```python
from build123d import *

# Parameters (mm, degrees)
SKETCH1_R           = 23
SKETCH1_R_2         = 14
BOSS_EXTRUDE1_DEPTH = 3.175


with BuildPart() as part:
    # Sketch1 → Boss-Extrude1 (new body)
    with BuildSketch(Plane(origin=(0, 0, 0), x_dir=(1, 0, 0), z_dir=(0, 1, 0))):
        Polygon((74.275, 82.5), (-74.275, 82.5), (-74.275, 76.15), (-144.275, 76.15), (-144.275, 82.5), (-225, 82.5), (-225, 35), (-218.65, 35), (-218.65, -35), (-225, -35), (-225, -82.5), (-165, -82.5), (-165, -76.15), (-95, -76.15), (-95, -82.5), (95, -82.5), (95, -76.15), (165, -76.15), (165, -82.5), (225, -82.5), (225, -35), (218.65, -35), (218.65, 35), (225, 35), (225, 82.5), (144.275, 82.5), (144.275, 76.15), (74.275, 76.15), align=None)
        with Locations(Location((-130, 37.5, 0), (0, 0, 270))):  # turned: the seam where the file's is
            Circle(SKETCH1_R, mode=Mode.SUBTRACT)
        with Locations(Location((-85, 0, 0), (0, 0, 270))):  # turned: the seam where the file's is
            Circle(SKETCH1_R, mode=Mode.SUBTRACT)
        with Locations(Location((-175, 0, 0), (0, 0, 270))):  # turned: the seam where the file's is
            Circle(SKETCH1_R, mode=Mode.SUBTRACT)
        with Locations(Location((-130, -37.5, 0), (0, 0, 270))):  # turned: the seam where the file's is
            Circle(SKETCH1_R, mode=Mode.SUBTRACT)
        with Locations(Location((130, 37.5, 0), (0, 0, 270))):  # turned: the seam where the file's is
            Circle(SKETCH1_R, mode=Mode.SUBTRACT)
        with Locations(Location((85, 0, 0), (0, 0, 270))):  # turned: the seam where the file's is
            Circle(SKETCH1_R, mode=Mode.SUBTRACT)
        with Locations(Location((175, 0, 0), (0, 0, 270))):  # turned: the seam where the file's is
            Circle(SKETCH1_R, mode=Mode.SUBTRACT)
        with Locations(Location((130, -37.5, 0), (0, 0, 270))):  # turned: the seam where the file's is
            Circle(SKETCH1_R, mode=Mode.SUBTRACT)
        with Locations(Location((-52.5, -57.5, 0), (0, 0, 270))):  # turned: the seam where the file's is
            Circle(SKETCH1_R_2, mode=Mode.SUBTRACT)
        with Locations(Location((-17.5, -57.5, 0), (0, 0, 270))):  # turned: the seam where the file's is
            Circle(SKETCH1_R_2, mode=Mode.SUBTRACT)
        with Locations(Location((17.5, -57.5, 0), (0, 0, 270))):  # turned: the seam where the file's is
            Circle(SKETCH1_R_2, mode=Mode.SUBTRACT)
        with Locations(Location((52.5, -57.5, 0), (0, 0, 270))):  # turned: the seam where the file's is
            Circle(SKETCH1_R_2, mode=Mode.SUBTRACT)
    extrude(amount=BOSS_EXTRUDE1_DEPTH)


solid = part.part
```
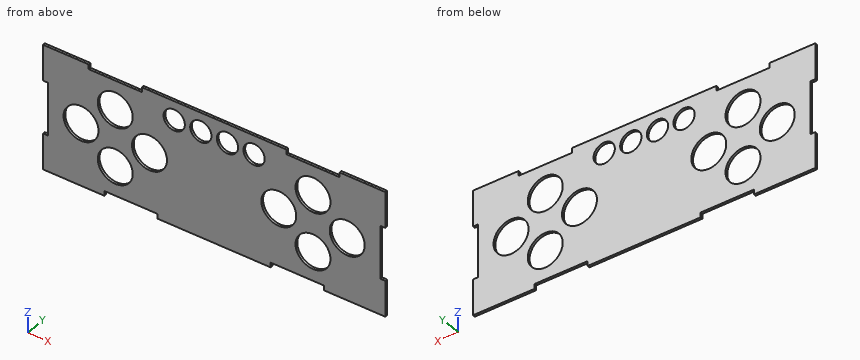
Read the model definition and answer for the solid it produces. Units are mm, in the model's axes. Coordinates: 2 decimals unless noted, no trailing zeros. Write each loop counter-clockwise with the first axis right and the second up, starting at its lowest first coordinate (ties: lowest second). Pieces come first, ordered by that corner, then holes. Notation, with made-up numbers: (29.5, -27.75) - (69.5, -27.75) arc R14 cw to (69.5, -21.75) - close; hole circle Ø5 at (58, 8.25). An arc over 180 degrees is marked (long way). Answer as a JSON object with one key per item and string values. Group by question number.
1. Consider L1, parallel to X at y = 1.6, z = 39; L2, parallel to Z at x = -121, y = 2.5; L3, parallel to X at y = 2.95, z = 14. Determine where each line is inside the solid, lowest interval first. Write a range as [from, to].
2. A cutting plane is placed at C-C (z = 48). Determine the outline of the cut face in (x, y) (3 decimals).
3. Each of these flat-tipped pins is pushed along its axis until it touches: P1, Ø1, axis at x = -115.5, y = 2, coming from the -Z side; P2, Ø8, axis at x = 131, z = -63, coming from the -Y side. Where does it stop, or does it pass through?
4. A cutting plane is placed at B-B (z = 5). Determine the outline of the cut face in (x, y) (3 decimals).
5. A cutting plane is placed at A-A (x = 17.5). Determine the outline of the cut face in (y, z) (3 decimals), plus the area to 3 significant figures.
6. A cutting plane is placed at D-D (x = -175). Determine the outline of the cut face in (y, z) (3 decimals).
Worked out:
{
 "1": {"L1": "x = [-225, -152.95], [-107.05, 107.05], [152.95, 225]", "L2": "z = [-76.15, -58.67], [-16.33, 16.33], [58.67, 76.15]", "L3": "x = [-218.65, -193.25], [-156.75, -103.25], [-66.75, 66.75], [103.25, 156.75], [193.25, 218.65]"},
 "2": {"outline": "(-225, 0) - (-150.463, 0) - (-150.463, 3.175) - (-225, 3.175) - close; (-109.537, 0) - (-62.783, 0) - (-62.783, 3.175) - (-109.537, 3.175) - close; (-42.217, 0) - (-27.783, 0) - (-27.783, 3.175) - (-42.217, 3.175) - close; (-7.217, 0) - (7.217, 0) - (7.217, 3.175) - (-7.217, 3.175) - close; (27.783, 0) - (42.217, 0) - (42.217, 3.175) - (27.783, 3.175) - close; (62.783, 0) - (109.537, 0) - (109.537, 3.175) - (62.783, 3.175) - close; (150.463, 0) - (225, 0) - (225, 3.175) - (150.463, 3.175) - close"},
 "3": {"P1": "stops at z = -76.15", "P2": "stops at y = 0"},
 "4": {"outline": "(-218.65, 0) - (-197.45, 0) - (-197.45, 3.175) - (-218.65, 3.175) - close; (-152.55, 0) - (-107.45, 0) - (-107.45, 3.175) - (-152.55, 3.175) - close; (-62.55, 0) - (62.55, 0) - (62.55, 3.175) - (-62.55, 3.175) - close; (107.45, 0) - (152.55, 0) - (152.55, 3.175) - (107.45, 3.175) - close; (197.45, 0) - (218.65, 0) - (218.65, 3.175) - (197.45, 3.175) - close"},
 "5": {"outline": "(0, -82.5) - (3.175, -82.5) - (3.175, 43.5) - (0, 43.5) - close; (0, 71.5) - (3.175, 71.5) - (3.175, 82.5) - (0, 82.5) - close", "area": "435 mm²"},
 "6": {"outline": "(0, -82.5) - (3.175, -82.5) - (3.175, -23) - (0, -23) - close; (0, 23) - (3.175, 23) - (3.175, 82.5) - (0, 82.5) - close"}
}
